Could you check a few things on this model? Use its own coordinates, in mm. A direction names the side the tool comes from. Round coordinates to 2 decimals unless told otherwise and drop trailing zeros. Write each loop counter-clockwise with the first axis right and the second up, starting at its lowest first coordinate (ties: lowest second). Pieces come first, ordered by that corner, then holes.
```python
from build123d import *

# Parameters (mm, degrees)
F1_DEPTH = 20
F2_R     = 3.25
F3_DEPTH = 20.001


with BuildPart() as f1:
    # F0 (on Top) → F1 (new body)
    with BuildSketch(Plane.XY):
        with BuildLine():
            Line((-5.2141973622, 0.6), (-60, 0.6))
            Line((-60, 0.6), (-60, -0.6))
            Line((-60, -0.6), (-5.2141973622, -0.6))
            ThreePointArc((-5.2141973622, -0.6), (-5.2486049701, 0), (-5.2141973622, 0.6))
        make_face()
        with BuildLine():
            ThreePointArc((-3.1267139234, 4.215627376), (-4.5454252385, 2.624302485), (-5.2141973622, 0.6))
            Line((-5.2141973622, 0.6), (-1.0392304845, 0.6))
            Line((-1.0392304845, 0.6), (-3.1267139234, 4.215627376))
        make_face()
        with BuildLine():
            Line((-1.0392304845, 0.6), (-5.2141973622, 0.6))
            ThreePointArc((-5.2141973622, 0.6), (-5.2486049701, 0), (-5.2141973622, -0.6))
            Line((-5.2141973622, -0.6), (-1.0392304845, -0.6))
            Line((-1.0392304845, -0.6), (-0.692820323, 0))
            Line((-0.692820323, 0), (-1.0392304845, 0.6))
        make_face()
        with BuildLine():
            Line((-3.1267139234, 4.215627376), (-1.0392304845, 0.6))
            Line((-1.0392304845, 0.6), (-0.3464101615, 0.6))
            Line((-0.3464101615, 0.6), (0, 1.2))
            Line((0, 1.2), (-2.0874834388, 4.815627376))
            ThreePointArc((-2.0874834388, 4.815627376), (-2.624302485, 4.5454252385), (-3.1267139234, 4.215627376))
        make_face()
        with BuildLine():
            Line((-30.5196152423, 51.6615242271), (-3.1267139234, 4.215627376))
            ThreePointArc((-3.1267139234, 4.215627376), (-2.624302485, 4.5454252385), (-2.0874834388, 4.815627376))
            Line((-2.0874834388, 4.815627376), (-29.4803847577, 52.2615242271))
            Line((-29.4803847577, 52.2615242271), (-30.5196152423, 51.6615242271))
        make_face()
        with BuildLine():
            Line((-1.0392304845, -0.6), (-5.2141973622, -0.6))
            ThreePointArc((-5.2141973622, -0.6), (-4.5454252385, -2.624302485), (-3.1267139234, -4.215627376))
            Line((-3.1267139234, -4.215627376), (-1.0392304845, -0.6))
        make_face()
        with BuildLine():
            ThreePointArc((2.0874834388, 4.815627376), (0, 5.2486049701), (-2.0874834388, 4.815627376))
            Line((-2.0874834388, 4.815627376), (0, 1.2))
            Line((0, 1.2), (2.0874834388, 4.815627376))
        make_face()
        with BuildLine():
            Line((-0.3464101615, -0.6), (-1.0392304845, -0.6))
            Line((-1.0392304845, -0.6), (-3.1267139234, -4.215627376))
            ThreePointArc((-3.1267139234, -4.215627376), (-2.624302485, -4.5454252385), (-2.0874834388, -4.815627376))
            Line((-2.0874834388, -4.815627376), (0, -1.2))
            Line((0, -1.2), (-0.3464101615, -0.6))
        make_face()
        with BuildLine():
            ThreePointArc((-2.0874834388, -4.815627376), (-2.624302485, -4.5454252385), (-3.1267139234, -4.215627376))
            Line((-3.1267139234, -4.215627376), (-30.5196152423, -51.6615242271))
            Line((-30.5196152423, -51.6615242271), (-29.4803847577, -52.2615242271))
            Line((-29.4803847577, -52.2615242271), (-2.0874834388, -4.815627376))
        make_face()
        with BuildLine():
            Line((2.0874834388, 4.815627376), (0, 1.2))
            Line((0, 1.2), (0.3464101615, 0.6))
            Line((0.3464101615, 0.6), (1.0392304845, 0.6))
            Line((1.0392304845, 0.6), (3.1267139234, 4.215627376))
            ThreePointArc((3.1267139234, 4.215627376), (2.624302485, 4.5454252385), (2.0874834388, 4.815627376))
        make_face()
        with BuildLine():
            Line((29.4803847577, 52.2615242271), (2.0874834388, 4.815627376))
            ThreePointArc((2.0874834388, 4.815627376), (2.624302485, 4.5454252385), (3.1267139234, 4.215627376))
            Line((3.1267139234, 4.215627376), (30.5196152423, 51.6615242271))
            Line((30.5196152423, 51.6615242271), (29.4803847577, 52.2615242271))
        make_face()
        with BuildLine():
            Line((0, -1.2), (-2.0874834388, -4.815627376))
            ThreePointArc((-2.0874834388, -4.815627376), (0, -5.2486049701), (2.0874834388, -4.815627376))
            Line((2.0874834388, -4.815627376), (0, -1.2))
        make_face()
        with BuildLine():
            ThreePointArc((5.2141973622, 0.6), (4.5454252385, 2.624302485), (3.1267139234, 4.215627376))
            Line((3.1267139234, 4.215627376), (1.0392304845, 0.6))
            Line((1.0392304845, 0.6), (5.2141973622, 0.6))
        make_face()
        with BuildLine():
            Line((0.3464101615, -0.6), (0, -1.2))
            Line((0, -1.2), (2.0874834388, -4.815627376))
            ThreePointArc((2.0874834388, -4.815627376), (2.624302485, -4.5454252385), (3.1267139234, -4.215627376))
            Line((3.1267139234, -4.215627376), (1.0392304845, -0.6))
            Line((1.0392304845, -0.6), (0.3464101615, -0.6))
        make_face()
        with BuildLine():
            ThreePointArc((3.1267139234, -4.215627376), (2.624302485, -4.5454252385), (2.0874834388, -4.815627376))
            Line((2.0874834388, -4.815627376), (29.4803847577, -52.2615242271))
            Line((29.4803847577, -52.2615242271), (30.5196152423, -51.6615242271))
            Line((30.5196152423, -51.6615242271), (3.1267139234, -4.215627376))
        make_face()
        with BuildLine():
            Line((5.2141973622, 0.6), (1.0392304845, 0.6))
            Line((1.0392304845, 0.6), (0.692820323, 0))
            Line((0.692820323, 0), (1.0392304845, -0.6))
            Line((1.0392304845, -0.6), (5.2141973622, -0.6))
            ThreePointArc((5.2141973622, -0.6), (5.2399960077, -0.3004928799), (5.2486049701, 0))
            ThreePointArc((5.2486049701, 0), (5.2399960077, 0.3004928799), (5.2141973622, 0.6))
        make_face()
        with BuildLine():
            Line((60, 0.6), (5.2141973622, 0.6))
            ThreePointArc((5.2141973622, 0.6), (5.2399960077, 0.3004928799), (5.2486049701, 0))
            ThreePointArc((5.2486049701, 0), (5.2399960077, -0.3004928799), (5.2141973622, -0.6))
            Line((5.2141973622, -0.6), (60, -0.6))
            Line((60, -0.6), (60, 0.6))
        make_face()
        with BuildLine():
            Line((1.0392304845, -0.6), (3.1267139234, -4.215627376))
            ThreePointArc((3.1267139234, -4.215627376), (4.5454252385, -2.624302485), (5.2141973622, -0.6))
            Line((5.2141973622, -0.6), (1.0392304845, -0.6))
        make_face()
    extrude(amount=F1_DEPTH)

    # F2 (on face) → F3 (cut, through all)
    with BuildSketch(Plane.XY.offset(20)):
        Circle(F2_R)
        Polygon((1.0392304845, 0.6), (0.692820323, 0), (1.0392304845, -0.6), (0.3464101615, -0.6), (0, -1.2), (-0.3464101615, -0.6), (-1.0392304845, -0.6), (-0.692820323, 0), (-1.0392304845, 0.6), (-0.3464101615, 0.6), (0, 1.2), (0.3464101615, 0.6), align=None, mode=Mode.SUBTRACT)
    extrude(amount=-F3_DEPTH, mode=Mode.SUBTRACT)


solid = f1.part
```
Q1. On a 3-axis mill with a long thin cutter (end or side, diameter ignored), from which of +Z, -Z, +X, -X, +Y, -Y can I reach the whole of each face in a straight line? I mean faces 1 (the flat face through (0, -4, 20)), 2 (the flat face through (-32, 0.6, 10)), 3 (the flat face through (16.631, 27.606, 9.86)), 4 (the flat face through (15.592, -28.206, 9.86)), 5 (the flat face through (15.976, 28.871, 9.86)). Say none if no direction works.
Q2. Imagine slicing it at D-D, the plane x = 22. Write out the boundary of the cut face in (y, z).
Q3. We'd pull the mould along Y, two halves only. Please class faces 6 (the cylindrical face through (4.56, 2.6, 9.86)), 7 (the cylindrical face through (0.03, 5.25, 9.86)), 8 (the flat face through (-17.015, 28.271, 9.86)), 9 (the cylindrical face through (-0.03, -5.25, 9.86)): pulls with the +Y half, pulls with the -Y half, needs draft (parallel to the pull), parting line crosses it, or undercut.
Q4. I'm going to push flat-ended pins straight in: pin 1 Ø6 at (x, z) = (-47.5, 5.5) entering from +Y; pin 2 Ø10 at (x, z) = (22, 7) entering from -Y; pin 3 Ø4 at (x, y) = (0, 0) entering from +Z; pin 4 Ø8 at (y, z) = (36.5, 14) entering from +X. Where does each tip first touch, or does it pass through?
Q5. If I drill on L1, parallel to Y at x = -21, z = 13.75; L2, parallel to X at y = 11.5, z = 4.75; L3, parallel to Y at x = -54, z = 11.25, over which ranges is the centre line in solid material (lowest first)?
Q6. Imagine slicing it at C-C, the plane y = -11. Write out the boundary of the cut face in (x, z), then the cut area to 3 significant figures.
Q7. Imagine slicing it at B-B, the plane z = 13. Write out the boundary of the cut face in (x, y), then the cut area to 3 significant figures.
Q8. Imagine slicing it at A-A, the plane x = 0. Write out the boundary of the cut face in (y, z), then the cut area to 3 significant figures.
Results found:
1. face 1: +Z, +X, -X, +Y, -Y
1. face 2: +Z, -Z, -X
1. face 3: +Z, -Z, +X
1. face 4: +Z, -Z, -Y
1. face 5: +Z, -Z, +Y
2. outline: (-39.31, 0) - (-36.91, 0) - (-36.91, 20) - (-39.31, 20) - close; (-0.6, 0) - (0.6, 0) - (0.6, 20) - (-0.6, 20) - close; (36.91, 0) - (39.31, 0) - (39.31, 20) - (36.91, 20) - close
3. face 6: undercut
3. face 7: pulls with the +Y half
3. face 8: undercut
3. face 9: pulls with the -Y half
4. pin 1: stops at y = 0.6
4. pin 2: stops at y = -47.97
4. pin 3: passes through
4. pin 4: stops at x = 24.08
5. L1: y = -37.57 to -35.17, -0.6 to 0.6, 35.17 to 37.57
5. L2: x = -7.33 to -5.95, 5.95 to 7.33
5. L3: y = -0.6 to 0.6
6. outline: (-7.04, 0) - (-5.66, 0) - (-5.66, 20) - (-7.04, 20) - close; (5.66, 0) - (7.04, 0) - (7.04, 20) - (5.66, 20) - close
6. area: 55.4 mm2
7. outline: (-60, -0.6) - (-5.21, -0.6) arc R5.25 ccw to (-3.13, -4.22) - (-30.52, -51.66) - (-29.48, -52.26) - (-2.09, -4.82) arc R5.25 ccw to (2.09, -4.82) - (29.48, -52.26) - (30.52, -51.66) - (3.13, -4.22) arc R5.25 ccw to (5.21, -0.6) - (60, -0.6) - (60, 0.6) - (5.21, 0.6) arc R5.25 ccw to (3.13, 4.22) - (30.52, 51.66) - (29.48, 52.26) - (2.09, 4.82) arc R5.25 ccw to (-2.09, 4.82) - (-29.48, 52.26) - (-30.52, 51.66) - (-3.13, 4.22) arc R5.25 ccw to (-5.21, 0.6) - (-60, 0.6) - close; hole circle Ø6.5 at (0, 0)
7. area: 448 mm2
8. outline: (-5.25, 0) - (-3.25, 0) - (-3.25, 20) - (-5.25, 20) - close; (3.25, 0) - (5.25, 0) - (5.25, 20) - (3.25, 20) - close
8. area: 79.9 mm2
